For this review, take the finished solid that the model builds, in its own axes (mm). Face numbers are marked on the shaded views. A direction names the side the tool comes from. Coordinates: 2 decimals unless noted, no trailing zeros. Order: outer loops, then holes, each group sorted by start corner. A loop starts at its lowest first (then second) coordinate and runs counter-clockwise, first axis right, second up. Notation, with made-up numbers: (12, 22.25) -> (65, 22.25) arc R11 ccw to (65, 29.25) -> close; hole circle Ø5 at (82.25, 48.5). An arc over 180 degrees is marked (long way). Answer as a JSON object with one key per item and string values. Group by question number.
1) Draft analysis for pull direction Y (two halves, no side actions). For the marked faces 1, 2, 3 and 4, state which applies: +Y half, -Y half, draft (parallel to the pull), parting line (faces both ways), or undercut.
2) Wall thickness on L1, parallel to X at y = 5.5, z = 5.5; L2, parallel to Z at x = -1.5, y = 6.5; L3, parallel to Z at x = -5, y = 5: over which ranges is each line inside the solid? List them lowest first.
3) Add section B-B, the plane z = 3.75. Write out the cut boundary in (x, y).
4) Add section C-C, the plane y = -7.25. Write out the cut boundary in (x, z).
5) Add section A-A, the plane x = 5. Write out the cut boundary in (y, z).
6) For pin 1 (1.1 mm diameter, centred on y = 5.5, z = -6.5, fed in from +X); pin 2 (1 mm diameter, centred on x = -3.5, y = 2, fed in from +Z); pin 3 (0.8 mm diameter, centred on x = -14.5, y = -8.5, fed in from -Z), all flat-tipped, find the tip position at first contact; note any pin that passes through.
7) Add section D-D, the plane x = 10.5. Write out the cut boundary in (y, z), then the cut area to 3 significant figures.
8) Machinability: for the marked faces 5, 6 and 7, which of the approach directions +Z, -Z, +X, -X, +Y, -Y give a long, thin tool a straight path to every point of the face, cutting with its end or side? Answer none if there is none.
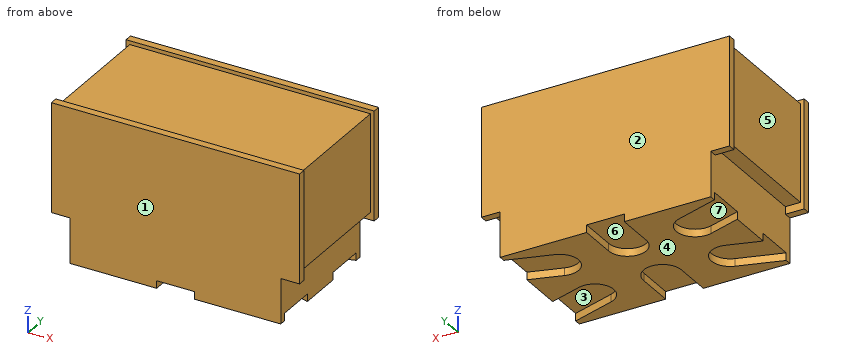
Autodesk Inventor part; units mm, degrees
ref_plane "Work Plane1" through (-16, 0, 13) normal (0, 1, 0) x (1, 0, 0)
ref_plane "YZ Plane" through (0, 0, 0) normal (1, 0, 0) x (0, 1, 0)
ref_plane "XZ Plane" through (0, 0, 0) normal (0, 1, 0) x (-1, 0, 0)
sketch "Sketch1" plane through (0, 0, 0) normal (0, 0, 1) x (1, 0, 0)
  line L0 (-16, -8) -> (16, -8)
  line L1 (16, -8) -> (16, 8)
  line L2 (16, 8) -> (-16, 8)
  line L3 (-16, 8) -> (-16, -8)
  point P0 (0, 0)
  point P1 (0, 8)
  point P2 (16, 0)
  dimension "d0" = 32
  dimension "d1" = 16
extrude "Extrusion1" add sketch "Sketch1" along normal blind 13
sketch "Sketch2" plane through (-16, -8, 0) normal (0, -1, 0) x (1, 0, 0)
  line L0 (32, 13) -> (0, 13)
  line L1 (0, 0) -> (0, 13)
  line L2 (0, 0) -> (32, 0)
  line L3 (32, 0) -> (32, 13)
  line L4 (-1, 14) -> (33, 14)
  line L5 (33, 14) -> (33, -1)
  line L6 (33, -1) -> (-1, -1)
  line L7 (-1, -1) -> (-1, 14)
  line L8 (2, -1) -> (30, -1)
  line L9 (30, -1) -> (30, -7)
  line L10 (30, -7) -> (2, -7)
  line L11 (2, -7) -> (2, -1)
  point P0 (16, 0)
  dimension "d4" = 1
  dimension "d5" = 3
  dimension "d6" = 3
  dimension "d7" = 6
extrude "Extrusion2" add sketch "Sketch2" along normal blind 1 contours L3 L2 L1 L0 | L4 L5 L6 L7 | L6 L9 L10 L11
sketch "Sketch3" plane through (-16, -8, 0) normal (0, 1, 0) x (1, 0, 0)
  line L0 (0, 0) -> (32, 0)
  line L1 (2, 7) -> (30, 7)
  line L2 (30, 7) -> (30, 0)
  line L3 (30, 0) -> (2, 0)
  line L4 (2, 0) -> (2, 7)
  point P0 (16, 0)
extrude "Extrusion3" add sketch "Sketch3" along normal up to surface (16 mm away)
sketch "Sketch4" plane through (-16, 8, 13) normal (0, 1, 0) x (1, 0, 0)
  line L0 (0, 0) -> (32, 0)
  line L1 (32, 13) -> (32, 0)
  line L2 (32, 13) -> (30, 13)
  line L3 (30, 20) -> (30, 13)
  line L4 (2, 20) -> (30, 20)
  line L5 (2, 13) -> (2, 20)
  line L6 (2, 13) -> (0, 13)
  line L7 (0, 13) -> (0, 0)
  line L8 (-1, 14) -> (2, 14)
  line L9 (2, 13) -> (2, 14)
  line L10 (-1, 14) -> (2, 14)
  line L11 (-1, -1) -> (-1, 14)
  line L12 (33, -1) -> (-1, -1)
  line L13 (33, 14) -> (33, -1)
  line L14 (30, 14) -> (33, 14)
  line L15 (30, 14) -> (30, 13)
  line L16 (30, 13) -> (32, 13)
  line L17 (32, 13) -> (32, 0)
  line L18 (32, 0) -> (0, 0)
  line L19 (0, 13) -> (0, 0)
  line L20 (0, 13) -> (2, 13)
  point P0 (16, 13)
extrude "Extrusion4" add sketch "Sketch4" along normal blind 1
sketch "Sketch5" plane through (14, -9, -7) normal (0, 0, -1) x (-1, 0, 0)
  line L0 (28, 0) -> (28, 18)
  line L1 (28, 18) -> (0, 18)
  line L2 (0, 18) -> (0, 0)
  line L3 (11.5, 18) -> (16.5, 18)
  line L4 (16.5, 18) -> (16.5, 13)
  line L5 (16.5, 13) -> (11.5, 13)
  line L6 (11.5, 13) -> (11.5, 18)
  circle A0 centre (14, 13) radius 2.5
  circle A1 centre (23, 13) radius 2.5
  line L7 (23.7463, 10.614) -> (28, 11.9446)
  line L8 (22.2537, 15.386) -> (28, 17.1835)
  circle A2 centre (5, 13) radius 2.5
  line L9 (4.2537, 10.614) -> (0, 11.9446)
  line L10 (5.7463, 15.386) -> (0, 17.1835)
  point P0 (14, 9)
  point P1 (14, 18)
  point P2 (14, 18)
  dimension "d14" = 5
  dimension "d15" = 5
  dimension "d16" = 5
  dimension "d17" = 9
  dimension "d18" = 5
  dimension "d19" = 9
extrude "Extrusion5" cut sketch "Sketch5" against normal blind 1
ref_plane "Work Plane1" through (-16, 0, 13) normal (0, 1, 0) x (1, 0, 0)
mirror "Mirror1" about plane through (-16, 0, 13) normal (0, 1, 0) of "Extrusion5"
sketch "Sketch6" plane through (-17, -8, 14) normal (0, 0, 1) x (1, 0, 0)
  line L0 (0, -1) -> (34, -1)
  line L1 (34, 0) -> (34, -1)
  line L2 (34, 0) -> (0, 0)
  line L3 (0, 0) -> (0, -1)
  line L4 (34, 17) -> (0, 17)
  line L5 (0, 16) -> (0, 17)
  line L6 (0, 16) -> (34, 16)
  line L7 (34, 16) -> (34, 17)
  point P0 (17, 8)
extrude "Extrusion6" cut sketch "Sketch6" against normal blind 0.5
sketch "Sketch7" plane through (17, -9, -1) normal (1, 0, 0) x (0, 0, -1)
  line L0 (-14.5, 1) -> (-14.5, 0)
  line L1 (-14.5, 0) -> (0, 0)
  line L2 (0, 1) -> (0, 0)
  line L3 (0, 1) -> (-14.5, 1)
  line L4 (-14.5, 18) -> (-14.5, 17)
  line L5 (-14.5, 17) -> (0, 17)
  line L6 (0, 17) -> (0, 18)
  line L7 (0, 18) -> (-14.5, 18)
  point P0 (-1, 9)
extrude "Extrusion7" cut sketch "Sketch7" against normal blind 0.5
sketch "Sketch8" plane through (-17, 8, -1) normal (-1, 0, 0) x (0, 0, 1)
  line L0 (14.5, 0) -> (14.5, 1)
  line L1 (14.5, 1) -> (0, 1)
  line L2 (0, 0) -> (0, 1)
  line L3 (0, 0) -> (14.5, 0)
  line L4 (14.5, -17) -> (14.5, -16)
  line L5 (14.5, -16) -> (0, -16)
  line L6 (0, -16) -> (0, -17)
  line L7 (0, -17) -> (14.5, -17)
  point P0 (1, -8)
extrude "Extrusion8" cut sketch "Sketch8" against normal blind 0.5
equation "\"d6\" = d5"
properties part number "03"
Output values:
{
 "1": {"face 1": "-Y half", "face 2": "+Y half", "face 3": "undercut", "face 4": "draft"},
 "2": {"L1": "x = -16 to 16", "L2": "z = -6 to 13", "L3": "z = -7 to 13"},
 "3": {"outline": "(-16.5, -9) -> (16.5, -9) -> (16.5, -8) -> (16, -8) -> (16, 8) -> (16.5, 8) -> (16.5, 9) -> (-16.5, 9) -> (-16.5, 8) -> (-16, 8) -> (-16, -8) -> (-16.5, -8) -> close"},
 "4": {"outline": "(-16, 0) -> (-14, 0) -> (-14, -6) -> (-11.02, -6) -> (-11.02, -7) -> (-2.5, -7) -> (-2.5, -6) -> (2.5, -6) -> (2.5, -7) -> (11.02, -7) -> (11.02, -6) -> (14, -6) -> (14, 0) -> (16, 0) -> (16, 13) -> (-16, 13) -> close"},
 "5": {"outline": "(-9, -7) -> (9, -7) -> (9, 13.5) -> (8, 13.5) -> (8, 13) -> (-8, 13) -> (-8, 13.5) -> (-9, 13.5) -> close"},
 "6": {"pin 1": "stops at x = 14", "pin 2": "stops at z = 13", "pin 3": "stops at z = -1"},
 "7": {"outline": "(-9, -7) -> (-7.09, -7) -> (-7.09, -6) -> (-1.85, -6) -> (-1.85, -7) -> (1.85, -7) -> (1.85, -6) -> (7.09, -6) -> (7.09, -7) -> (9, -7) -> (9, 13.5) -> (8, 13.5) -> (8, 13) -> (-8, 13) -> (-8, 13.5) -> (-9, 13.5) -> close", "area": "351 mm²"},
 "8": {"face 5": "+Z, -Z, -X", "face 6": "-Z, +Y", "face 7": "-Z"}
}
